Verification items for the finished model (mm, model axes). Face numbers are marked on the shaded views. A direction names the side the tool comes from. Give positions to 0.01 mm unless a question says otherwise; leave off trailing zeros. Loops run counter-clockwise (first coordinate to the right, second up) from the corner with the lowest first, then second, coordinate; pieces in that order, holes last. Notation, with made-up numbers: M -32,-31.75 L -10,-31.75 A20 ccw -10,-26.75 Z; hole C 3.5,4 d3. An arc over 180 degrees is marked long. Answer in a Markdown table with one row per item.
Solid Edge part; units mm, degrees
sketch "Sketch1" plane through (0, 0, 0) normal (0, -1, 0) x (1, 0, 0)
  line L0 (-50.5, 14.32) -> (-50.5, -5.68)
  line L1 (-50.5, -5.68) -> (-47.5, -5.68)
  line L2 (-47.5, -5.68) -> (-47.5, 4.32)
  line L3 (-47.5, 4.32) -> (-39.5, 4.32)
  line L4 (-39.5, 4.32) -> (-39.5, -5.68)
  line L5 (-39.5, -5.68) -> (-37, -5.68)
  line L6 (-37, -5.68) -> (-37, 5.7972)
  line L7 (-37, 5.7972) -> (0, 20)
  line L8 (0, 20) -> (0, 0)
  line L9 (0, 0) -> (4, 0)
  line L10 (4, 0) -> (4, 20)
  line L11 (4, 20) -> (21.44, 21.017)
  arc A0 (21.44, 21.017) -> (17.2742, 40.3358) centre (20.8579, 31) ccw
  line L12 (17.2742, 40.3358) -> (-50.5, 14.32)
  circle A1 centre (20.8579, 31) radius 5.5
  dimension "D1" = 50.5
  dimension "D2" = 39.5
  dimension "D3" = 47.5
  dimension "D4" = 4
  dimension "D5" = 50.5
  dimension "D6" = 20.8579
  dimension "D7" = 37
  dimension "D8" = 50.5
extrude "Protrusion1" add sketch "Sketch1" along normal blind 10
sketch "Sketch2" plane through (0, 0, 0) normal (0, -1, 0) x (1, 0, 0)
  line L0 (4, 20) -> (4, 0)
  line L1 (4, 20) -> (21.44, 21.017)
  line L2 (4.0411, 0) -> (27.935, 23.935)
  arc A0 (21.44, 21.017) -> (27.935, 23.935) centre (20.8579, 31) ccw
extrude "ProtrusiónExtruida_2" add sketch "Sketch2" along normal blind 2 material side at (4.05, 0, 10)
fillet "Redondeo_1" radius 5 4 edges at (-49, -10, -5.68) (-38.25, -10, -5.68) (-38.25, 0, -5.68) (-49, 0, -5.68)
fillet "Redondeo_2" radius 2 2 edges at (2, -10, 0) (2, 0, 0)
hole "Agujero_1" at (-50.5, -5, -0.68) direction (1, 0, 0) diameter 5.3 depth 31.9512
sketch "Sketch3" plane through (4, -6, 10) normal (1, 0, 0) x (0, 1, 0)
  circle A0 centre (1, -10) radius 1.5
extrude "Cutout1" cut sketch "Sketch3" against normal up to next
hole "Agujero_3" at (4, -5, 7.7972) direction (-1, 0, 0) diameter 1 end up to next
hole "Hole1" at (4, -5, 9.7972) direction (-1, 0, 0) diameter 1 end up to next
hole "Hole2" at (4, -5, 11.7972) direction (-1, 0, 0) diameter 1 end up to next
hole "Hole3" at (4, -5, 5.7972) direction (-1, 0, 0) diameter 1 end up to next
hole "Hole4" at (4, -5, 3.7972) direction (-1, 0, 0) diameter 1 end up to next
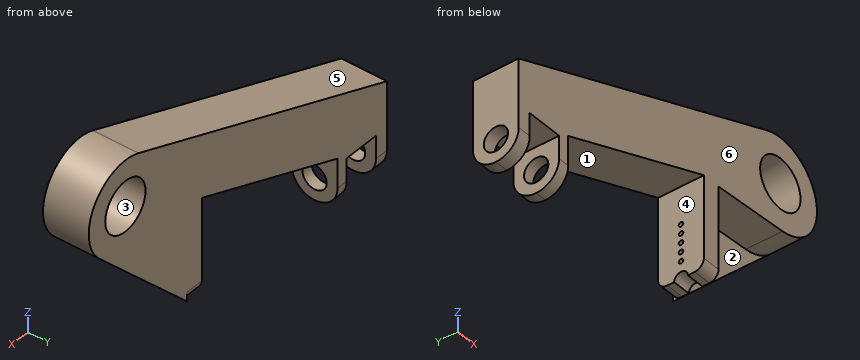
Item 1: Tool access check on the marked faces 1, 2 and 3. Record the directions out of +Z, -Z, +X, -X, +Y, -Y that give a thin tool (end or side, any length) a straight path to the whole face; none if there is none.
Reported:
| item | result |
|---|---|
| face 1 | -Z, +Y, -Y |
| face 2 | -Z, +X, -Y |
| face 3 | +Y, -Y |
Item 2: Scan lines: L1, parallel to Z at x = 2.75, y = -5; L2, parallel to Z at x = 1.7, y = -5; L3, parallel to Z at x = -48.9, y = -5. Record each from-to range of solid material in increasing order. Write a range as [from, to].
Reported:
| item | result |
|---|---|
| L1 | z = [1.5, 3.3], [4.3, 5.3], [6.3, 7.3], [8.3, 9.3], [10.3, 11.3], [12.3, 34.76] |
| L2 | z = [1.5, 3.3], [4.3, 5.3], [6.3, 7.3], [8.3, 9.3], [10.3, 11.3], [12.3, 34.36] |
| L3 | z = [-5.68, -3.33], [1.97, 14.93] |
Item 3: Go/stop test with flat-tipped pins: pin 1 (0.8 mm diameter, centred on x = 2, y = -7.5, fed in from -Z); pin 2 (2 mm diameter, centred on y = -5, z = 34.5, fed in from +X); pin 3 (3 mm diameter, centred on y = -5, z = -0.68, fed in from +X); pin 4 (5 mm diameter, centred on y = -5, z = -0.68, fed in from -X). Record where each tip stops, or that it passes through.
Reported:
| item | result |
|---|---|
| pin 1 | stops at z = 0 |
| pin 2 | stops at x = 30.54 |
| pin 3 | passes through |
| pin 4 | stops at x = 0 |
Item 4: Sectioned sample at A-A (y = -9). Record the cut outline in (x, z).
Reported:
| item | result |
|---|---|
| outline | M -50.5,-3.68 L -47.5,-3.68 L -47.5,4.32 L -39.5,4.32 L -39.5,-3.68 L -37,-3.68 L -37,5.8 L 0,20 L 0,0.27 L 4,0.27 L 4,20 L 21.44,21.02 A10 ccw long 17.27,40.34 L -50.5,14.32 Z; hole C 20.86,31 d11 |
Item 5: Release check for a two-part mould opening along X. For the marked faces 4, 5 and 6 record: released by +X, released by -X, zero draft, split by the parting line, or undercut.
Reported:
| item | result |
|---|---|
| face 4 | undercut |
| face 5 | released by -X |
| face 6 | zero draft |
Item 6: Sectioned sample at B-B (x = 23.5). Record the cut outline in (y, z).
Reported:
| item | result |
|---|---|
| outline | M -10,21.36 L -2,21.36 L -2,19.49 L 0,19.49 L 0,26.18 L -10,26.18 Z; M -10,35.82 L 0,35.82 L 0,40.64 L -10,40.64 Z |
Item 7: Sectioned sample at D-D (y = -1). Record the cut outline in (x, z).
Reported:
| item | result |
|---|---|
| outline | M -50.5,-3.68 L -47.5,-3.68 L -47.5,4.32 L -39.5,4.32 L -39.5,-3.68 L -37,-3.68 L -37,5.8 L 0,20 L 0,0.27 L 4,0.27 L 4,-0.04 L 27.94,23.93 A10 ccw 17.27,40.34 L -50.5,14.32 Z; hole C 20.86,31 d11 |
Item 8: Sectioned sample at C-C (z = 32). Record the cut outline in (x, y), and give its area (3 significant figures).
Reported:
| item | result |
|---|---|
| outline | M -4.44,-10 L 15.45,-10 L 15.45,0 L -4.44,0 Z; M 26.27,-10 L 30.81,-10 L 30.81,0 L 26.27,0 Z |
| area | 244 mm^2 |
